Source: CAD feature listing. Evaluate the final solid. Frame: model axes, mm. A direction names the side the tool comes from. Give positions to 0.01 mm unless a question says otherwise; leave off trailing zeros. Order: outer loops, then holes, each group sorted by start corner. A loop starts at its lowest first (then second) coordinate and runs counter-clockwise, first axis right, second up. Notation, with made-up numbers: (16, -20.5) - (75, -20.5) arc R22 cw to (75, -6.5) - close; hole circle Ø6 at (-8.75, 43.25). An arc over 180 degrees is marked (long way). Write each question's results on one line, items separated by ' | '. Start each with the question number.
Item 1: Line query: line 1 along X through (y, z) = (-30, -1.75); line 2 along X through (y, z) = (-30, -8.4); line 3 along X through (y, z) = (-25, -1.5). Output: solid intervals per line, ascending.
Item 2: Contact query for a flat-ended pin moving along its axis: pin 1 Ø11.5 at (x, y) = (-13, -30) entering from -Z. Output: stop coordinate, or through.
Item 3: Mould query, pull axis Y, two halves, no side actions, for faces 1 (the flat face through (-15, -33, -5.4)), 2 (the flat face through (-1, 110, -7)), 3 (the flat face through (-33, 2, 10)). Classes: released by +Y, released by -Y, zero draft, split by the parting line, or undercut.
Item 4: Section C-C on x = 13. Output: boundary loops of the cut face in (y, z).
Item 5: Section B-B on y = -30. Output: boundary loops of the cut face in (x, z), and give its area (3 significant figures).
Item 6: Set-up query: faces 4 (the flat face through (-8, -2, 0)), 5 (the cylindrical face through (-9.7, -30.1, 2.4)), 6 (the flat face through (-5, -2, 7)), 7 (the flat face through (15, -33, -5.4)). Return all of +Z, -Z, +X, -X, +Y, -Y with unobstructed straight access to the full face (end or side cutting, diameter ignored); none if empty.
Item 7: Section A-A on z = 1.25. Output: boundary loops of the cut face in (x, y), and give its area (3 significant figures).
```python
from build123d import *

# Parameters (mm, degrees)
F0_W           = 120
F0_H           = 220
F1_DEPTH       = 10
F3_DEPTH       = 220.001
F4_SIZE        = 3
F6_D           = 6.6
F6_CBORE_D     = 13
F6_CBORE_DEPTH = 4.6


# Not quite as in the source:
# - a pattern or mirror of a feature is missing from the dataset's text; its kind, count and spacing are read off the source's solid


with BuildPart() as f1:
    # F0 (on Top) → F1 (new body, symmetric)
    with BuildSketch(Plane.XY):
        Rectangle(F0_W, F0_H)
    extrude(amount=F1_DEPTH, both=True)

    # F2 (on face) → F3 (cut, through all)
    with BuildSketch(Plane.XZ.offset(110)):
        Polygon((5, 10), (-5, 10), (-5, 3.5), (-8, 3.5), (-8, -4.5), (8, -4.5), (8, 3.5), (5, 3.5), align=None)
    extrude(amount=-F3_DEPTH, mode=Mode.SUBTRACT)

    # F4
    f4_edges = [f1.edges().sort_by_distance(p)[0] for p in [
        (60, -110, 0),
        (60, 110, 0),
        (-60, 110, 0),
        (-60, -110, 0),
    ]]
    chamfer(f4_edges, length=F4_SIZE)

    # F6 (through all)
    with Locations(Plane(origin=(0, 0, -10), x_dir=(1, 0, 0), z_dir=(0, 0, -1))):
        with Locations((-13, 30)):
            f6 = CounterBoreHole(F6_D / 2, F6_CBORE_D / 2, F6_CBORE_DEPTH)

    # F6_copies: F6 across plane
    add(f6.mirror(Plane(origin=(0, 0, 0), x_dir=(0, 0, 1), z_dir=(1, 0, 0))), mode=Mode.SUBTRACT)


solid = f1.part
```
Evaluation:
1) line 1: x = -60 to -16.3, -9.7 to -8, 8 to 9.7, 16.3 to 60 | line 2: x = -60 to -19.5, -6.5 to 6.5, 19.5 to 60 | line 3: x = -60 to -8, 8 to 60
2) pin 1: stops at z = -5.4
3) face 1: undercut | face 2: released by +Y | face 3: zero draft
4) outline: (-110, -10) - (-36.5, -10) - (-36.5, -5.4) - (-33.3, -5.4) - (-33.3, 10) - (-110, 10) - close; (-26.7, -5.4) - (-23.5, -5.4) - (-23.5, -10) - (110, -10) - (110, 10) - (-26.7, 10) - close
5) outline: (-60, -10) - (-19.5, -10) - (-19.5, -5.4) - (-16.3, -5.4) - (-16.3, 10) - (-60, 10) - close; (-9.7, -5.4) - (-6.5, -5.4) - (-6.5, -10) - (6.5, -10) - (6.5, -5.4) - (9.7, -5.4) - (9.7, 10) - (5, 10) - (5, 3.5) - (8, 3.5) - (8, -4.5) - (-8, -4.5) - (-8, 3.5) - (-5, 3.5) - (-5, 10) - (-9.7, 10) - close; (16.3, -5.4) - (19.5, -5.4) - (19.5, -10) - (60, -10) - (60, 10) - (16.3, 10) - close | area: 1,880 mm^2
6) face 4: +Y, -Y | face 5: +Z, -Z | face 6: +Z, +Y, -Y | face 7: -Z
7) outline: (-60, -107) - (-57, -110) - (-8, -110) - (-8, 110) - (-57, 110) - (-60, 107) - close; (8, -110) - (57, -110) - (60, -107) - (60, 107) - (57, 110) - (8, 110) - close; hole circle Ø6.6 at (-13, -30); hole circle Ø6.6 at (13, -30) | area: 22,800 mm^2
